Input: dimensioned drawing with shaded views. Units: mm. Origin: part minimum x, y, z. Round coordinates to 2 decimals unless told otherwise and drop trailing zeros. Order: outer loops, then holes, each group sorted by start corner. A loop starts at its lowest first (then second) coordinate and runs counter-clockwise, first axis right, second up. Notation, with made-up numbers: M 22.5,26 L 29.5,26 A30 cw 29.5,52 Z; hole C 59.25,-19 d5. An arc over 180 degrees is marked long. Answer as CSV lines item,"result". Start each with the question number.
Item 1: Section query A-A on z = 28.75. Return the cut outline in (x, y) (3 decimals), plus the area to 4 significant figures.
Item 2: Section query D-D on z = 3. Return the cut outline in (x, y).
Item 3: Section query C-C on y = 0.7. Return the cut outline in (x, z) (3 decimals), plus the area to 3 significant figures.
Item 4: Section query B-B on x = 57.5. Return the cut outline in (y, z) (3 decimals).
Item 5: Line query: line 1 (Z direction, x = 57.5, y = 0.8) (3 decimals); line 2 (Z direction, x = 7, y = 0.85); line 3 (X direction, y = 0.4, z = 7). Output: solid intervals per line, ascending. Write a range as [from, to].
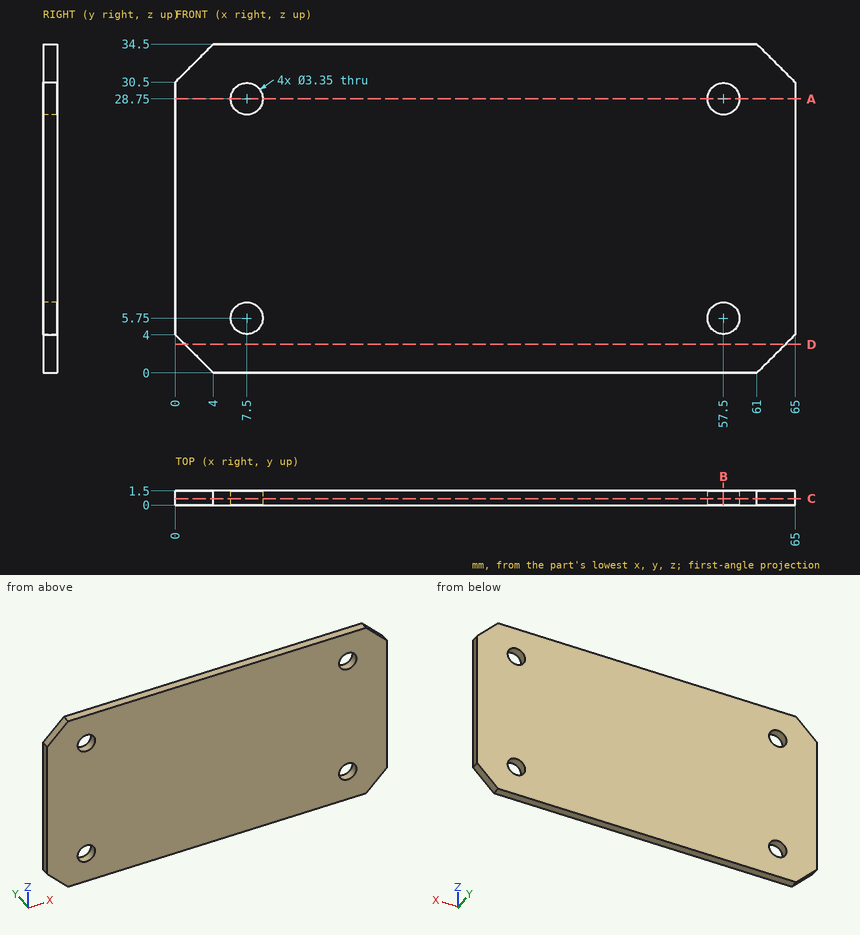
Results:
1,outline,"M 0,0 L 5.825,0 L 5.825,1.5 L 0,1.5 Z; M 9.175,0 L 55.825,0 L 55.825,1.5 L 9.175,1.5 Z; M 59.175,0 L 65,0 L 65,1.5 L 59.175,1.5 Z"
1,area,"87.45 mm^2"
2,outline,"M 1,0 L 64,0 L 64,1.5 L 1,1.5 Z"
3,outline,"M 0,4 L 4,0 L 61,0 L 65,4 L 65,30.5 L 61,34.5 L 4,34.5 L 0,30.5 Z; hole C 7.5,5.75 d3.35; hole C 7.5,28.75 d3.35; hole C 57.5,5.75 d3.35; hole C 57.5,28.75 d3.35"
3,area,"2,180 mm^2"
4,outline,"M 0,0 L 1.5,0 L 1.5,4.075 L 0,4.075 Z; M 0,7.425 L 1.5,7.425 L 1.5,27.075 L 0,27.075 Z; M 0,30.425 L 1.5,30.425 L 1.5,34.5 L 0,34.5 Z"
5,line 1,"[0, 4.075], [7.425, 27.075], [30.425, 34.5]"
5,line 2,"[0, 4.15], [7.35, 27.15], [30.35, 34.5]"
5,line 3,"[0, 6.39], [8.61, 56.39], [58.61, 65]"
